Answer from the drawing. Dimensions are ordinates in mm from the lowest x, y and z of the part. Coordinates: 2 decimals unless noted, no trailing zeros. Loops run counter-clockwise (first coordinate to the right, second up) from the corner with the lowest first, then second, coordinate; pieces in that order, holes last. Notation, with made-up numbers: (78.5, -35.5) - (106.5, -35.5) arc R20 cw to (106.5, -8.5) - close; hole circle Ø4 at (88, -15). An arc over 180 degrees is marked (long way). Write each question's results on one line, items separated by ' | '. Start each with the question number.
1. Each of these flat-tipped pins is pushed along its axis until it touches: P1, Ø1.5, axis at x = 13.5, z = 125.5, coming from the +Y side; P2, Ø3, axis at x = 11.5, y = 2, coming from the +Z side; P3, Ø1.5, axis at y = 11.5, z = 65, coming from the -X side. Where does it stop, or does it pass through?
2. A cutting plane is placed at B-B on z = 68. Determine the outline of the cut face in (x, y).
3. A cutting plane is placed at C-C on y = 14. Determine the outline of the cut face in (x, z), then the cut area to 3 significant figures.
4. A cutting plane is placed at D-D on x = 5. Determine the outline of the cut face in (y, z), then the cut area to 3 significant figures.
5. A cutting plane is placed at A-A on x = 10. Determine the outline of the cut face in (y, z).
6. Find the intervals of material crossed by line 1 along Z through (x, y) = (15.25, 1.75); line 2 along X through (y, z) = (10.25, 100.5); line 3 along X through (y, z) = (4, 11.5), in increasing order. Write a range as [from, to].
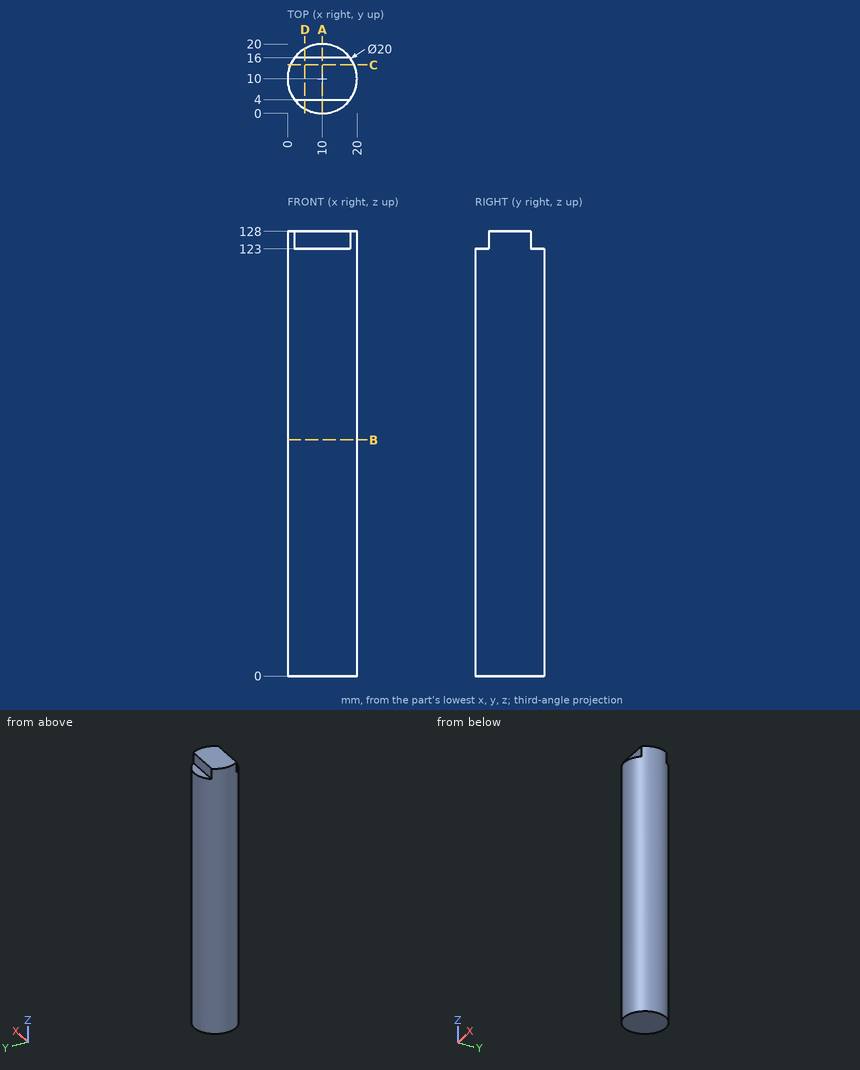
Values:
1) P1: y = 16 | P2: z = 123 | P3: x = 0.03
2) outline: circle Ø20 at (10, 10)
3) outline: (0.83, 0) - (19.17, 0) - (19.17, 128) - (0.83, 128) - close | area: 2,350 mm^2
4) outline: (1.34, 0) - (18.66, 0) - (18.66, 123) - (16, 123) - (16, 128) - (4, 128) - (4, 123) - (1.34, 123) - close | area: 2,190 mm^2
5) outline: (0, 0) - (20, 0) - (20, 123) - (16, 123) - (16, 128) - (4, 128) - (4, 123) - (0, 123) - close
6) line 1: [0, 123] | line 2: [0, 20] | line 3: [2, 18]
